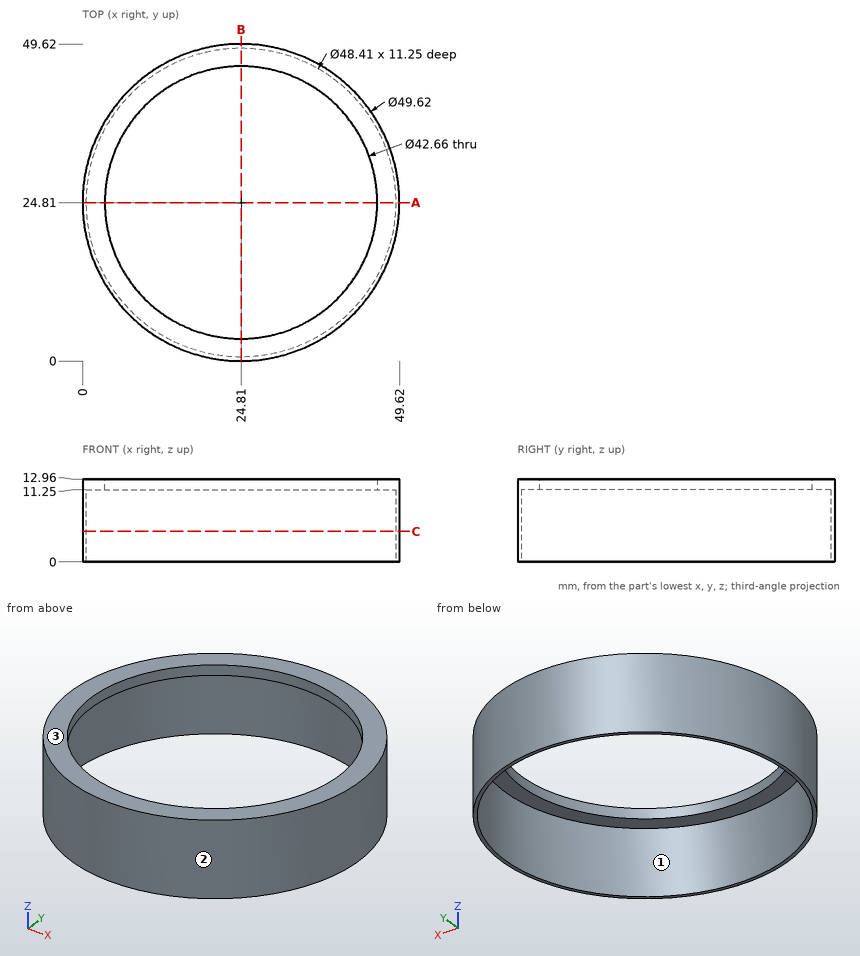
Print and shaded views of the part. All mm, measured from the part's lowest x, y and z. Give positions to 0.01 mm unless a question says otherwise; leave off trailing zeros. Write each loop counter-clockwise with the first axis right and the second up, starting at its lowest first coordinate (ties: lowest second). Pieces come first, ordered by that corner, then holes. Notation, with made-up numbers: (19, -37.5) -> (27, -37.5) arc R20 ccw to (27, -5.5) -> close; hole circle Ø8 at (-13.5, 64.5). An arc over 180 degrees is marked (long way). Write item = value, one per line.
(1) Flat gauge pins, fed straight in: P1, Ø1.5, axis at x = 7.5, y = 35.5, coming from the +Z side (3 decimals); P2, Ø2, axis at x = 32, z = 8.5, coming from the -Y side; P3, Ø2, axis at x = 33.5, z = 11.5, coming from the +Y side; P4, Ø1.5, axis at y = 44.5, z = 9, coming from the -X side. Where does each tip first touch, or does it go through?
Determined:
P1 = through
P2 = 0.78
P3 = 48.4
P4 = 8.78
(2) Mould opens along X. For the marked faces 1, 2 and 3 say: released by +X, released by -X, zero draft, split by the parting line, or undercut.
Determined:
face_1 = undercut
face_2 = split by the parting line
face_3 = zero draft
(3) Slice it at A-A, the plane y = 24.81. Give the cut face in (x, z) (3 decimals).
Determined:
outline = (0, 0) -> (0.605, 0) -> (0.605, 11.25) -> (3.48, 11.25) -> (3.48, 12.96) -> (0, 12.96) -> close; (46.14, 11.25) -> (49.015, 11.25) -> (49.015, 0) -> (49.62, 0) -> (49.62, 12.96) -> (46.14, 12.96) -> close
(4) Slice it at C-C, the plane z = 4.75. Give the cut face in (x, y) (3 decimals).
Determined:
outline = circle Ø49.62 at (24.81, 24.81); hole circle Ø48.41 at (24.81, 24.81)
(5) Probe line 1 along Y through (x, z) = (24.81, 3.5) (3 decimals); line 2 along X through (y, z) = (24.5, 11.5); line 3 along Z through (x, y) = (10.5, 8). List the from-to ranges inside material, lowest first.
Determined:
line_1 = 0 to 0.605, 49.015 to 49.62
line_2 = 0 to 3.48, 46.14 to 49.62
line_3 = 11.25 to 12.96
